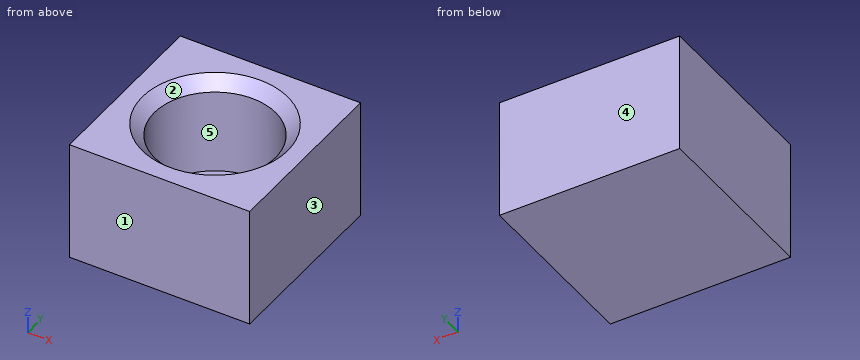
Autodesk Fusion 360 part; units mm, degrees
sketch "Sketch1" plane through (0, 0, 0) normal (0, 0, 1) x (1, 0, 0)
  line L0 (-19.05, -19.05) -> (19.05, -19.05)
  line L1 (19.05, -19.05) -> (19.05, 19.05)
  line L2 (19.05, 19.05) -> (-19.05, 19.05)
  line L3 (-19.05, 19.05) -> (-19.05, -19.05)
  line L4 (0, 1.75) -> (0, 22.5)
  line L5 (1.75, 0) -> (22.5, 0)
  dimension "d1" = 38.1
  dimension "d2" = 38.1
extrude "Extrude1" add sketch "Sketch1" along normal blind 25.4
sketch "Sketch2" plane through (0, 0, 25.4) normal (0, 0, 1) x (-1, 0, 0)
  line L0 (19.05, -19.05) -> (19.05, 19.05)
  line L1 (19.05, 19.05) -> (-19.05, 19.05)
  line L2 (-19.05, 19.05) -> (-19.05, -19.05)
  line L3 (-19.05, -19.05) -> (19.05, -19.05)
  circle A0 centre (0, 0) radius 12.827
  dimension "d5" = 25.654
extrude "Extrude2" cut sketch "Sketch2" against normal blind 20.32 contours A0
chamfer "Chamfer2" distance 2.54 angle 45 1 edges at (11.959, -4.6384, 25.4)
Check sheet for the modelled part. Datum: model origin and axes. Units: mm. Face numbers are marked on the shaded views. A direction names the side the tool comes from. Round coordinates to 2 decimals unless told otherwise and drop trailing zeros. Loops run counter-clockwise (first coordinate to the right, second up) from the corner with the lowest first, then second, coordinate; pieces in that order, holes last. Notation, with made-up numbers: M -17,-8.75 L 11,-8.75 A21 cw 11,21.25 Z; hole C 33.5,86 d3. An arc over 180 degrees is marked long. Answer as a JSON object with one key per item and string values.
1. Section check B-B (x = 0). Record the boundary of the cut face in (y, z), plus the area to 3 significant figures.
Reply:
{"outline": "M -19.05,0 L 19.05,0 L 19.05,25.4 L 15.37,25.4 L 12.83,22.86 L 12.83,5.08 L -12.83,5.08 L -12.83,22.86 L -15.37,25.4 L -19.05,25.4 Z", "area": "440 mm²"}
2. Mould release check, pull along X, two halves, no side actions. Record for the marked faces 1, 2 and 3: pulls with the +X half, pulls with the -X half, needs draft (parallel to the pull), parting line crosses it, or undercut.
Reply:
{"face 1": "needs draft", "face 2": "undercut", "face 3": "pulls with the +X half"}
3. Section check A-A (z = 7.25). Record the boundary of the cut face in (x, y).
Reply:
{"outline": "M -19.05,-19.05 L 19.05,-19.05 L 19.05,19.05 L -19.05,19.05 Z; hole C 0,0 d25.65"}
4. Scan lines: line 1 (Y direction, x = 0, z = 11.25); line 2 (X direction, y = -0.5, z = 24). Record each from-to range of solid material in increasing order.
Reply:
{"line 1": "y = -19.05 to -12.83, 12.83 to 19.05", "line 2": "x = -19.05 to -13.96, 13.96 to 19.05"}
5. Access from +Z, -Z, +X, -X, +Y, -Y to the whole of each face (thin tool, end or side, straight path). Record for the marked faces 4 and 5.
Reply:
{"face 4": "+Z, -Z, +X, -X, +Y", "face 5": "+Z"}
6. Gauge pin test, flat ends, axial feed: P1, Ø1.5, axis at x = 11.5, y = -7.5, coming from the +Z side; P2, Ø2, axis at x = 1.5, y = 8, coming from the +Z side. Record the tip position at first contact, or that the pin passes through.
Reply:
{"P1": "stops at z = 24.51", "P2": "stops at z = 5.08"}
